from build123d import *

# Parameters (mm, degrees)
F0_W     = 135.382
F0_H     = 78.994
F0_R     = 2.7178
F0_R_2   = 1.7272
F0_R_3   = 0.3175
F1_DEPTH = 4.699
F3_DEPTH = 3.0226


with BuildPart() as f1:
    # F0 (on Top) → F1 (new body)
    with BuildSketch(Plane.XY):
        Rectangle(F0_W, F0_H)
        with Locations((-38.2016, -28.067)):
            Circle(F0_R, mode=Mode.SUBTRACT)
        with Locations((-19.685, -28.067)):
            Circle(F0_R_2, mode=Mode.SUBTRACT)
        with Locations((-0.381, -28.067)):
            Circle(F0_R, mode=Mode.SUBTRACT)
        with Locations((37.9476, -28.067)):
            Circle(F0_R, mode=Mode.SUBTRACT)
        with Locations((-62.103, 1.143)):
            Circle(F0_R, mode=Mode.SUBTRACT)
        with Locations((-18.796, 4.953)):
            Circle(F0_R_3, mode=Mode.SUBTRACT)
        with Locations((-16.2052, 4.953)):
            Circle(F0_R_3, mode=Mode.SUBTRACT)
        with Locations((-13.6144, 4.953)):
            Circle(F0_R_3, mode=Mode.SUBTRACT)
        with Locations((-11.0236, 4.953)):
            Circle(F0_R_3, mode=Mode.SUBTRACT)
        with Locations((-8.4328, 4.953)):
            Circle(F0_R_3, mode=Mode.SUBTRACT)
        with Locations((-5.842, 4.953)):
            Circle(F0_R_3, mode=Mode.SUBTRACT)
        with Locations((-3.2512, 4.953)):
            Circle(F0_R_3, mode=Mode.SUBTRACT)
        with Locations((-0.6604, 4.953)):
            Circle(F0_R_3, mode=Mode.SUBTRACT)
        with BuildLine():
            ThreePointArc((-23.6093, 31.115), (-21.364236, 30.185064), (-20.4343, 27.94))
            Line((-20.4343, 27.94), (-20.4343, 4.826))
            ThreePointArc((-20.4343, 4.826), (-21.364236, 2.580936), (-23.6093, 1.651))
            ThreePointArc((-23.6093, 1.651), (-25.854364, 2.580936), (-26.7843, 4.826))
            Line((-26.7843, 4.826), (-26.7843, 27.94))
            ThreePointArc((-26.7843, 27.94), (-25.854364, 30.185064), (-23.6093, 31.115))
        make_face(mode=Mode.SUBTRACT)
        with Locations((-62.103, 26.543)):
            Circle(F0_R, mode=Mode.SUBTRACT)
        with Locations((-18.796, 27.813)):
            Circle(F0_R_3, mode=Mode.SUBTRACT)
        with Locations((-16.2052, 27.813)):
            Circle(F0_R_3, mode=Mode.SUBTRACT)
        with Locations((-13.6144, 27.813)):
            Circle(F0_R_3, mode=Mode.SUBTRACT)
        with Locations((-11.0236, 27.813)):
            Circle(F0_R_3, mode=Mode.SUBTRACT)
        with Locations((-8.4328, 27.813)):
            Circle(F0_R_3, mode=Mode.SUBTRACT)
        with Locations((-5.842, 27.813)):
            Circle(F0_R_3, mode=Mode.SUBTRACT)
        with Locations((-3.2512, 27.813)):
            Circle(F0_R_3, mode=Mode.SUBTRACT)
        with Locations((-0.6604, 27.813)):
            Circle(F0_R_3, mode=Mode.SUBTRACT)
        with Locations((1.9304, 4.953)):
            Circle(F0_R_3, mode=Mode.SUBTRACT)
        with Locations((4.5212, 4.953)):
            Circle(F0_R_3, mode=Mode.SUBTRACT)
        with BuildLine():
            Line((6.0579, 4.826), (6.0579, 27.94))
            ThreePointArc((6.0579, 27.94), (6.987836, 30.185064), (9.2329, 31.115))
            ThreePointArc((9.2329, 31.115), (11.477964, 30.185064), (12.4079, 27.94))
            Line((12.4079, 27.94), (12.4079, 4.826))
            ThreePointArc((12.4079, 4.826), (11.477964, 2.580936), (9.2329, 1.651))
            ThreePointArc((9.2329, 1.651), (6.987836, 2.580936), (6.0579, 4.826))
        make_face(mode=Mode.SUBTRACT)
        with Locations((62.103, 1.143)):
            Circle(F0_R, mode=Mode.SUBTRACT)
        with Locations((1.9304, 27.813)):
            Circle(F0_R_3, mode=Mode.SUBTRACT)
        with Locations((4.5212, 27.813)):
            Circle(F0_R_3, mode=Mode.SUBTRACT)
        with Locations((62.103, 26.543)):
            Circle(F0_R, mode=Mode.SUBTRACT)
    extrude(amount=F1_DEPTH)

    # F2 (on face) → F3 (cut)
    with BuildSketch(Plane.XY.offset(4.699)):
        with BuildLine():
            Line((29.083, 39.497), (-32.131, 39.497))
            Line((-32.131, 39.497), (-32.131, 0.635))
            ThreePointArc((-32.131, 0.635), (-31.015077, -2.059077), (-28.321, -3.175))
            Line((-28.321, -3.175), (25.273, -3.175))
            ThreePointArc((25.273, -3.175), (27.967077, -2.059077), (29.083, 0.635))
            Line((29.083, 0.635), (29.083, 39.497))
        make_face()
    extrude(amount=-F3_DEPTH, mode=Mode.SUBTRACT)


solid = f1.part
Geometry: final body of the model. Coordinates: model frame, mm. A direction names the side the tool comes from. Round coordinates to 2 decimals unless told otherwise and drop trailing zeros. Order: outer loops, then holes, each group sorted by start corner. A loop starts at its lowest first (then second) coordinate and runs counter-clockwise, first axis right, second up.
Q1. Pin query (flat end, axial travel): pin 1 (21.5 mm diameter, centred on x = 10, y = 12, fed in from +Z); pin 2 (2.5 mm diameter, centred on x = 9.5, z = 3, fed in from +Y) (3 decimals). Return the tip coordinate at first contact, or that it passes through.
Result sheet:
pin 1: stops at z = 1.68
pin 2: stops at y = -3.175
Q2. Section A-A, the plane y = 14. Output: boundary loops of the cut face in (x, z).
Result sheet:
outline: (-67.69, 0) - (-26.78, 0) - (-26.78, 1.68) - (-32.13, 1.68) - (-32.13, 4.7) - (-67.69, 4.7) - close; (-20.43, 0) - (6.06, 0) - (6.06, 1.68) - (-20.43, 1.68) - close; (12.41, 0) - (67.69, 0) - (67.69, 4.7) - (29.08, 4.7) - (29.08, 1.68) - (12.41, 1.68) - close
Q3. Section B-B, the plane x = -37. Output: boundary loops of the cut face in (y, z).
Result sheet:
outline: (-39.5, 0) - (-30.5, 0) - (-30.5, 4.7) - (-39.5, 4.7) - close; (-25.63, 0) - (39.5, 0) - (39.5, 4.7) - (-25.63, 4.7) - close
Q4. Access query for faces 1 (the face through (-59.51, 27.36, 2.32)), 2 (the face through (-2, 18, 1.676)). Directions: +Z, -Z, +X, -X, +Y, -Y. A direction counts if a zero-diameter tool reaches every point of the face in a straight line with its end or side. Return the directions, or none.
Result sheet:
face 1: +Z, -Z
face 2: +Z, +Y
Q5. Material intervals for probe 1 along X at (y, z) = (18, 0.5); probe 2 along X at (y, z) = (-1, 4.1); probe 3 along X at (y, z) = (29.5, 3.3), sorted ascending.
Result sheet:
probe 1: x = -67.69 to -26.78, -20.43 to 6.06, 12.41 to 67.69
probe 2: x = -67.69 to -63.77, -60.43 to -31.76, 28.71 to 60.43, 63.77 to 67.69
probe 3: x = -67.69 to -32.13, 29.08 to 67.69
Q6. Section C-C, the plane x = 19. Output: boundary loops of the cut face in (y, z) (3 decimals).
Result sheet:
outline: (-39.497, 0) - (39.497, 0) - (39.497, 1.676) - (-3.175, 1.676) - (-3.175, 4.699) - (-39.497, 4.699) - close
Q7. Section D-D, the plane z = 2.9. Give the number of separate pieces and of enclosed holes in the cut face, and give its area (3 significant figures).
Result sheet:
separate pieces: 1
enclosed holes: 8
area: 7,920 mm2
Q8. Mould query, pull axis X, two halves, no side actions, for faces 3 (the face through (-1, 1, 0)), 4 (the face through (-67.691, -1, 2)), 5 (the face through (-21.41, -27.99, 2.32)). Classes: released by +X, released by -X, zero draft, split by the parting line, or undercut.
Result sheet:
face 3: zero draft
face 4: released by -X
face 5: undercut
